Can you work these out from the drawing? Everything is in mm from the part's minimum corner. A direction names the side the tool comes from. Round coordinates to 2 decimals unless told otherwise and drop trailing zeros. Loops run counter-clockwise (first coordinate to the right, second up) from the corner with the lowest first, then second, coordinate; pieces in that order, holes last. Notation, with made-up numbers: (-34, 62) - (18, 62) arc R13 cw to (18, 71) - close; hole circle Ø8 at (-3, -33). An arc over 180 degrees is marked (long way). Answer as a JSON object with one key per item and string values. Group by question number.
1) I want a section at D-D, the plane y = 6. Please give me the cut outline in (x, z).
2) If I drill on line 1 along Y through (x, z) = (6.35, 1.65); line 2 along X through (y, z) = (1, 2.75); line 3 along Y through (x, z) = (30.5, 2), over which ranges is the centre line in solid material (lowest first)? Write a range as [from, to].
3) I want a section at A-A, the plane x = 6.35. Please give me the cut outline in (y, z).
4) I want a section at B-B, the plane y = 10. Please give me the cut outline in (x, z) (1 decimal), then the cut area to 3 significant figures.
5) Will these pins go through, and if not, where does the flat tip stop? P1, Ø1, axis at y = 5, z = 1, coming from the -X side; P2, Ø5, axis at x = 6.35, y = 9.575, coming from the +Z side; P3, Ø1.5, axis at y = 13.5, z = 1.5, coming from the +X side; P4, Ø0.9, axis at y = 2, z = 2, coming from the -X side.
6) Which directions (+Z, -Z, +X, -X, +Y, -Y) give clear straight access to the entire face, cutting with the end or side of a thin tool? Please do the marked faces 5, 6, 7 and 8.
7) If we mould it in two halves opening along Y, with no side actions, what happens to the marked faces 1, 2, 3 and 4? For each: pulls with the +Y half, pulls with the -Y half, needs draft (parallel to the pull), parting line crosses it, or undercut.
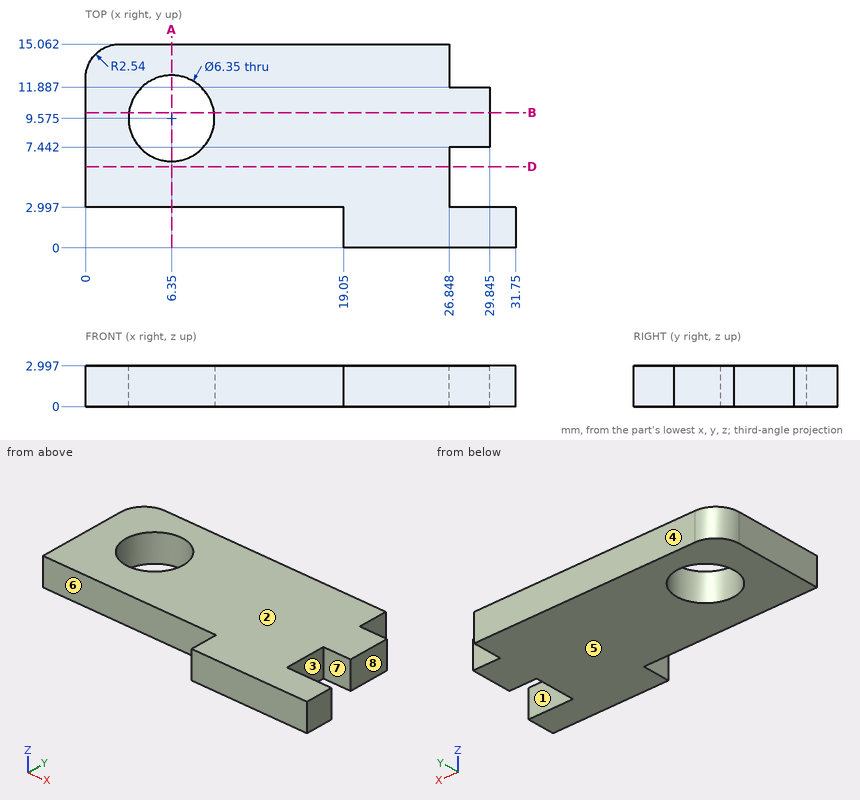
Outcome:
{
 "1": {"outline": "(0, 0) - (26.85, 0) - (26.85, 3) - (0, 3) - close"},
 "2": {"line 1": "[3, 6.4], [12.75, 15.06]", "line 2": "[19.05, 31.75]", "line 3": "[0, 3]"},
 "3": {"outline": "(3, 0) - (6.4, 0) - (6.4, 3) - (3, 3) - close; (12.75, 0) - (15.06, 0) - (15.06, 3) - (12.75, 3) - close"},
 "4": {"outline": "(0, 0) - (3.2, 0) - (3.2, 3) - (0, 3) - close; (9.5, 0) - (29.8, 0) - (29.8, 3) - (9.5, 3) - close", "area": "70.6 mm^2"},
 "5": {"P1": "x = 0", "P2": "through", "P3": "x = 26.85", "P4": "x = 19.05"},
 "6": {"face 5": "-Z, +X, -X, +Y, -Y", "face 6": "+Z, -Z, -X, -Y", "face 7": "+Z, -Z, +X", "face 8": "+Z, -Z, +X, +Y"},
 "7": {"face 1": "undercut", "face 2": "needs draft", "face 3": "undercut", "face 4": "pulls with the +Y half"}
}
